from build123d import *

# Parameters (mm, degrees)
SKETCH1_W           = 121.92
SKETCH1_H           = 66.04
BOSS_EXTRUDE1_DEPTH = 5.08
FILLET1_R           = 5.08
CUT_EXTRUDE2_REACH  = 140.75
SKETCH2_R           = 1.7526
SKETCH2_W           = 6.096
SKETCH2_H           = 12.446
SKETCH3_R           = 3.175
CUT_EXTRUDE3_DEPTH  = 3.81
CUT_EXTRUDE4_REACH  = 140.709
SKETCH4_R           = 1.9812
SKETCH8_W           = 15.24
SKETCH8_H           = 66.04
BOSS_EXTRUDE2_DEPTH = 5.08
FILLET4_R           = 5.08
SKETCH10_W          = 5.08
SKETCH10_H          = 25.4
BOSS_EXTRUDE4_DEPTH = 3.81
SKETCH11_W          = 50.8
SKETCH11_H          = 5.08
BOSS_EXTRUDE5_DEPTH = 3.81
FILLET5_R           = 5.08


with BuildPart() as part:
    # Sketch1 → Boss-Extrude1 (new body)
    with BuildSketch(Plane(origin=(0, 0, 0), x_dir=(1, 0, 0), z_dir=(0, 1, 0))):
        with Locations((60.96, 33.02)):
            Rectangle(SKETCH1_W, SKETCH1_H)
    extrude(amount=BOSS_EXTRUDE1_DEPTH)

    # Fillet1
    fillet1_edges = [part.edges().sort_by_distance(p)[0] for p in [
        (0, 2.54, -66.04),
        (121.92, 2.54, -66.04),
        (121.92, 2.54, 0),
        (0, 2.54, 0),
    ]]
    fillet(fillet1_edges, radius=FILLET1_R)

    # Sketch2 → Cut-Extrude2 (cut, up to next)
    with BuildSketch(Plane(origin=(0, 5.08, 0), x_dir=(1, 0, 0), z_dir=(0, 1, 0)), mode=Mode.PRIVATE) as cut_extrude2_sk1:
        with Locations(Location((30.48, 47.2694, 0), (0, 0, 270))):
            Circle(SKETCH2_R)
    cut_extrude2_tool1 = extrude(cut_extrude2_sk1.sketch, amount=-CUT_EXTRUDE2_REACH, mode=Mode.PRIVATE) & part.part
    # Sketch2 → Cut-Extrude2 (cut, up to next)
    with BuildSketch(Plane(origin=(0, 5.08, 0), x_dir=(1, 0, 0), z_dir=(0, 1, 0)), mode=Mode.PRIVATE) as cut_extrude2_sk2:
        with Locations(Location((30.48, 18.7706, 0), (0, 0, 90))):
            Circle(SKETCH2_R)
    cut_extrude2_tool2 = extrude(cut_extrude2_sk2.sketch, amount=-CUT_EXTRUDE2_REACH, mode=Mode.PRIVATE) & part.part
    # Sketch2 → Cut-Extrude2 (cut, up to next)
    with BuildSketch(Plane(origin=(0, 5.08, 0), x_dir=(1, 0, 0), z_dir=(0, 1, 0)), mode=Mode.PRIVATE) as cut_extrude2_sk3:
        with Locations((30.48, 33.02)):
            Rectangle(SKETCH2_W, SKETCH2_H)
    cut_extrude2_tool3 = extrude(cut_extrude2_sk3.sketch, amount=-CUT_EXTRUDE2_REACH, mode=Mode.PRIVATE) & part.part
    add(cut_extrude2_tool1.solids().sort_by_distance((30.48, 5.08, -47.2694))[0], mode=Mode.SUBTRACT)
    add(cut_extrude2_tool2.solids().sort_by_distance((30.48, 5.08, -18.7706))[0], mode=Mode.SUBTRACT)
    add(cut_extrude2_tool3.solids().sort_by_distance((30.48, 5.08, -33.02))[0], mode=Mode.SUBTRACT)

    # Sketch3 → Cut-Extrude3 (cut)
    with BuildSketch(Plane(origin=(0, 5.08, 0), x_dir=(1, 0, 0), z_dir=(0, 1, 0))):
        with Locations(Location((17.78, 40.64, 0), (0, 0, 270))):
            Circle(SKETCH3_R)
        with Locations(Location((17.78, 25.4, 0), (0, 0, 270))):
            Circle(SKETCH3_R)
    extrude(amount=-CUT_EXTRUDE3_DEPTH, mode=Mode.SUBTRACT)

    # Sketch4 → Cut-Extrude4 (cut, up to next)
    with BuildSketch(Plane(origin=(0, 1.27, 0), x_dir=(1, 0, 0), z_dir=(0, 1, 0)), mode=Mode.PRIVATE) as cut_extrude4_sk1:
        with Locations(Location((17.78, 40.64, 0), (0, 0, 270))):
            Circle(SKETCH4_R)
    cut_extrude4_tool1 = extrude(cut_extrude4_sk1.sketch, amount=-CUT_EXTRUDE4_REACH, mode=Mode.PRIVATE) & part.part
    # Sketch4 → Cut-Extrude4 (cut, up to next)
    with BuildSketch(Plane(origin=(0, 1.27, 0), x_dir=(1, 0, 0), z_dir=(0, 1, 0)), mode=Mode.PRIVATE) as cut_extrude4_sk2:
        with Locations(Location((17.78, 25.4, 0), (0, 0, 270))):
            Circle(SKETCH4_R)
    cut_extrude4_tool2 = extrude(cut_extrude4_sk2.sketch, amount=-CUT_EXTRUDE4_REACH, mode=Mode.PRIVATE) & part.part
    add(cut_extrude4_tool1.solids().sort_by_distance((17.78, 1.27, -40.64))[0], mode=Mode.SUBTRACT)
    add(cut_extrude4_tool2.solids().sort_by_distance((17.78, 1.27, -25.4))[0], mode=Mode.SUBTRACT)

    # Sketch8 → Boss-Extrude2 (add)
    with BuildSketch(Plane.XZ):
        with Locations((124.46, -33.02)):
            Rectangle(SKETCH8_W, SKETCH8_H)
    extrude(amount=-BOSS_EXTRUDE2_DEPTH)

    # Fillet4
    fillet4_edges = [part.edges().sort_by_distance(p)[0] for p in [
        (132.08, 2.54, 0),
        (132.08, 2.54, -66.04),
    ]]
    fillet(fillet4_edges, radius=FILLET4_R)

    # Sketch10 → Boss-Extrude4 (add)
    with BuildSketch(Plane(origin=(0, 5.08, 0), x_dir=(1, 0, 0), z_dir=(0, 1, 0))):
        with Locations((5.334, 33.02)):
            Rectangle(SKETCH10_W, SKETCH10_H)
        with Locations((126.746, 33.02)):
            Rectangle(SKETCH10_W, SKETCH10_H)
    extrude(amount=BOSS_EXTRUDE4_DEPTH)

    # Sketch11 → Boss-Extrude5 (add)
    with BuildSketch(Plane(origin=(0, 5.08, 0), x_dir=(1, 0, 0), z_dir=(0, 1, 0))):
        with Locations((66.04, 60.706)):
            Rectangle(SKETCH11_W, SKETCH11_H)
        with Locations((66.04, 5.334)):
            Rectangle(SKETCH11_W, SKETCH11_H)
    extrude(amount=BOSS_EXTRUDE5_DEPTH)

    # Fillet5
    fillet5_edges = [part.edges().sort_by_distance(p)[0] for p in [
        (40.64, 6.985, -7.874),
        (91.44, 6.985, -7.874),
        (124.206, 6.985, -20.32),
        (124.206, 6.985, -45.72),
        (91.44, 6.985, -58.166),
        (40.64, 6.985, -58.166),
        (7.874, 6.985, -20.32),
        (7.874, 6.985, -45.72),
    ]]
    fillet(fillet5_edges, radius=FILLET5_R - 0.0001)  # a hair under: the kernel refuses the full size


solid = part.part
Input: part model. Units: mm. Frame: model coordinates. A direction names the side the tool comes from. Coordinates: 2 decimals unless noted, no trailing zeros. Order: outer loops, then holes, each group sorted by start corner. A loop starts at its lowest first (then second) coordinate and runs counter-clockwise, first axis right, second up.
1. Access query for faces 5 (the cylindrical face through (125.7, 7, -21.8)), 6 (the cylindrical face through (89.9, 7, -59.6)), 7 (the flat face through (27.432, 3, -33)), 8 (the cylindrical face through (125.65, 7.01, -44.19)). Directions: +Z, -Z, +X, -X, +Y, -Y. A direction counts if a zero-diameter tool reaches every point of the face in a straight line with its end or side. Return the directions, or none.
Checked values:
face 5: +Z, +Y
face 6: +X, +Y
face 7: +Y, -Y
face 8: -Z, +Y
2. Ray query, line 1 along X through (y, z) = (3.8, -40.64) (3 decimals); line 2 along X through (y, z) = (1, -32); line 3 along Y through (x, z) = (123.5, -16). Return the intervals inside material, ascending.
Checked values:
line 1: x = 0 to 14.605, 20.955 to 132.08
line 2: x = 0 to 27.43, 33.53 to 132.08
line 3: y = 0 to 5.08
3. Draft query along X for faces 1 (the flat face through (132.08, 3, -33)), 2 (the flat face through (33.528, 3, -33)), 3 (the flat face through (127, 8.89, -33)), 4 (the cylindrical face through (15.846, 0.644, -41.069)). Return one class per face: +X half, -X half, draft (parallel to the pull), parting line (faces both ways), or undercut.
Checked values:
face 1: +X half
face 2: undercut
face 3: draft
face 4: undercut
4. Cut plane A-A, the plane z = -36. Return loops of the section in (x, y), plus the area to 3 significant figures.
Checked values:
outline: (0, 0) - (27.43, 0) - (27.43, 5.08) - (7.87, 5.08) - (7.87, 8.89) - (2.79, 8.89) - (2.79, 5.08) - (0, 5.08) - close; (33.53, 0) - (132.08, 0) - (132.08, 5.08) - (129.29, 5.08) - (129.29, 8.89) - (124.21, 8.89) - (124.21, 5.08) - (33.53, 5.08) - close
area: 679 mm2
5. Contact query for flat-ended pins moving along their axis: P1, Ø1.1, axis at y = 7, z = -32, coming from the -X side; P2, Ø8, axis at x = 50.5, z = -18.5, coming from the +Y side; P3, Ø4, axis at x = 60.5, y = 7.5, coming from the +Z side. Output: stop coordinate, or through.
Checked values:
P1: stops at x = 2.79
P2: stops at y = 5.08
P3: stops at z = -2.79
6. Cut plane D-D, the plane x = 69.5. Return loops of the section in (y, z).
Checked values:
outline: (0, -66.04) - (5.08, -66.04) - (5.08, -63.25) - (8.89, -63.25) - (8.89, -58.17) - (5.08, -58.17) - (5.08, -7.87) - (8.89, -7.87) - (8.89, -2.79) - (5.08, -2.79) - (5.08, 0) - (0, 0) - close
7. Cut plane C-C, the plane y = 3. Return loops of the section in (x, z) (3 decimals), plus the area to 3 significant figures.
Checked values:
outline: (0, -60.96) arc R5.08 ccw to (5.08, -66.04) - (127, -66.04) arc R5.08 ccw to (132.08, -60.96) - (132.08, -5.08) arc R5.08 ccw to (127, 0) - (5.08, 0) arc R5.08 ccw to (0, -5.08) - close; hole circle Ø6.35 at (17.78, -40.64); hole circle Ø6.35 at (17.78, -25.4); hole (27.432, -39.243) - (33.528, -39.243) - (33.528, -26.797) - (27.432, -26.797) - close; hole circle Ø3.505 at (30.48, -47.269); hole circle Ø3.505 at (30.48, -18.771)
area: 8,540 mm2
8. Cut plane B-B, the plane x = 17.78. Return loops of the section in (y, z) (3 decimals), plus the area to 3 significant figures.
Checked values:
outline: (0, -66.04) - (5.08, -66.04) - (5.08, -43.815) - (1.27, -43.815) - (1.27, -42.621) - (0, -42.621) - close; (0, -38.659) - (1.27, -38.659) - (1.27, -37.465) - (5.08, -37.465) - (5.08, -28.575) - (1.27, -28.575) - (1.27, -27.381) - (0, -27.381) - close; (0, -23.419) - (1.27, -23.419) - (1.27, -22.225) - (5.08, -22.225) - (5.08, 0) - (0, 0) - close
area: 277 mm2
